Input: part model. Units: mm. Frame: model coordinates. Face numbers are marked on the shaded views. Round coordinates to 2 decimals unless told otherwise and drop trailing zeros. Loops run counter-clockwise (first coordinate to the right, second up) from the corner with the lowest first, then second, coordinate; pieces in that order, holes last. Notation, with made-up numbers: M 74.25,-23 L 96.25,-23 A20 ccw 96.25,-18 Z; hole C -30.5,-18 d11. An arc over 180 degrees is marked long. Return JSON: item names as keys, results as strings. Group by question number.
1) Mould query, pull axis X, two halves, no side actions, for the marked faces 1, 2, 3 and 4. Classes: +X half, -X half, draft (parallel to the pull), parting line (faces both ways), or undercut.
2) Material intervals for line 1 (X direction, y = 33.5, z = 3.55); line 2 (X direction, y = 13, z = 3.85); line 3 (Y direction, x = 21.25, z = 3.2), sorted ascending. Write a range as from..to.
3) Section D-D (x = 15). Output: boundary loops of the cut face in (y, z).
4) Section B-B (y = 8.5). Output: boundary loops of the cut face in (x, z).
5) Section C-C (z = 0.65). Output: boundary loops of the cut face in (x, y).
6) Contact query for flat-ended pins moving along their axis: P1, Ø4, axis at x = 9.5, y = 8, coming from the +Z side; P2, Ø1, axis at y = 33.5, z = 4.5, coming from the +X side; P3, Ø1.3, axis at x = 9, z = 4.5, coming from the -Y side. Output: stop coordinate, or through.
7) Section A-A (x = 5). Output: boundary loops of the cut face in (y, z), plus the area to 3 significant figures.
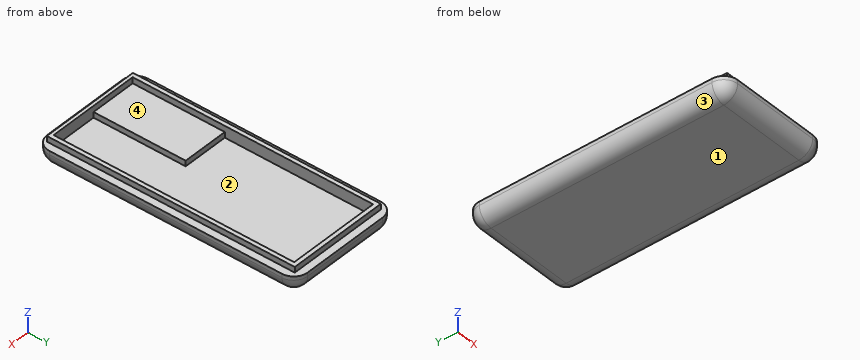
from build123d import *

# Parameters (mm, degrees)
SKETCH_1_W          = 25.2
SKETCH_1_H          = 56.5
EXTRUDE_1_DEPTH     = 5
SKETCH_2_W          = 25.2
SKETCH_2_H          = 56.5
SKETCH_2_W_2        = 22
SKETCH_2_H_2        = 53.8
CUT_EXTRUDE_1_DEPTH = 1.3
SKETCH_3_W          = 20.2
SKETCH_3_H          = 52.2
CUT_EXTRUDE_2_DEPTH = 2.6
SKETCH_4_W          = 0.1
SKETCH_4_H          = 53.8
CUT_EXTRUDE_3_DEPTH = 62.434599372
SKETCH_5_W          = 25.2
SKETCH_5_H          = 56.5
EXTRUDE_2_DEPTH     = 0.1
SKETCH_6_W          = 10
SKETCH_6_H          = 20
EXTRUDE_3_DEPTH     = 1.2
FILLET_1_R          = 3


with BuildPart() as part:
    # Эскиз1 → Бобышка-Вытянуть1 (new body)
    with BuildSketch(Plane.XY):
        with Locations((12.6, 28.25)):
            Rectangle(SKETCH_1_W, SKETCH_1_H)
    extrude(amount=EXTRUDE_1_DEPTH)

    # Эскиз2 → Вырез-Вытянуть1 (cut)
    with BuildSketch(Plane.XY.offset(5)):
        with Locations((12.6, 28.25)):
            Rectangle(SKETCH_2_W, SKETCH_2_H)
        with Locations((12.6, 28)):
            Rectangle(SKETCH_2_W_2, SKETCH_2_H_2, mode=Mode.SUBTRACT)
    extrude(amount=-CUT_EXTRUDE_1_DEPTH, mode=Mode.SUBTRACT)

    # Эскиз3 → Вырез-Вытянуть2 (cut)
    with BuildSketch(Plane.XY.offset(5)):
        with Locations((12.6, 27.9)):
            Rectangle(SKETCH_3_W, SKETCH_3_H)
    extrude(amount=-CUT_EXTRUDE_2_DEPTH, mode=Mode.SUBTRACT)

    # Эскиз4 → Вырез-Вытянуть3 (cut, through all)
    with BuildSketch(Plane.ZY.offset(-1.6)):
        with Locations((4.95, 28)):
            Rectangle(SKETCH_4_W, SKETCH_4_H)
    extrude(amount=-CUT_EXTRUDE_3_DEPTH, mode=Mode.SUBTRACT)

    # Эскиз5 → Бобышка-Вытянуть2 (add)
    with BuildSketch(Plane(origin=(0, 0, 0), x_dir=(-1, 0, 0), z_dir=(0, 0, -1))):
        with Locations((-12.6, 28.25)):
            Rectangle(SKETCH_5_W, SKETCH_5_H)
    extrude(amount=EXTRUDE_2_DEPTH)

    # Эскиз6 → Бобышка-Вытянуть3 (add)
    with BuildSketch(Plane.XY.offset(2.4)):
        with Locations((7.5, 11.8)):
            Rectangle(SKETCH_6_W, SKETCH_6_H)
    extrude(amount=EXTRUDE_3_DEPTH)

    # Скругление1
    fillet_1_edges = [part.edges().sort_by_distance(p)[0] for p in [
        (0, 56.5, 1.8),
        (25.2, 56.5, 1.8),
        (25.2, 0, 1.8),
        (0, 0, 1.8),
        (25.2, 28.25, -0.1),
        (12.6, 0, -0.1),
        (0, 28.25, -0.1),
        (12.6, 56.5, -0.1),
    ]]
    fillet(fillet_1_edges, radius=FILLET_1_R)


solid = part.part
Returned:
{
 "1": {"face 1": "draft", "face 2": "undercut", "face 3": "-X half", "face 4": "undercut"},
 "2": {"line 1": "x = 0..2.5, 22.7..25.2", "line 2": "x = 1.6..2.5, 22.7..23.6", "line 3": "y = 0..1.8, 54..56.5"},
 "3": {"outline": "M 0,2.9 A3 ccw 3,-0.1 L 53.5,-0.1 A3 ccw 56.5,2.9 L 56.5,3.7 L 54.9,3.7 L 54.9,4.9 L 54,4.9 L 54,2.4 L 1.8,2.4 L 1.8,4.9 L 1.1,4.9 L 1.1,3.7 L 0,3.7 Z"},
 "4": {"outline": "M 0,2.9 A3 ccw 3,-0.1 L 22.2,-0.1 A3 ccw 25.2,2.9 L 25.2,3.7 L 23.6,3.7 L 23.6,4.9 L 22.7,4.9 L 22.7,2.4 L 12.5,2.4 L 12.5,3.6 L 2.5,3.6 L 2.5,4.9 L 1.6,4.9 L 1.6,3.7 L 0,3.7 Z"},
 "5": {"outline": "M 1.02,3 A1.98 ccw 3,1.02 L 22.2,1.02 A1.98 ccw 24.18,3 L 24.18,53.5 A1.98 ccw 22.2,55.48 L 3,55.48 A1.98 ccw 1.02,53.5 Z"},
 "6": {"P1": "stops at z = 3.6", "P2": "stops at x = 23.6", "P3": "stops at y = 1.1"},
 "7": {"outline": "M 0,2.9 A3 ccw 3,-0.1 L 53.5,-0.1 A3 ccw 56.5,2.9 L 56.5,3.7 L 54.9,3.7 L 54.9,4.9 L 54,4.9 L 54,2.4 L 21.8,2.4 L 21.8,3.6 L 1.8,3.6 L 1.8,4.9 L 1.1,4.9 L 1.1,3.7 L 0,3.7 Z", "area": "169 mm^2"}
}
